from build123d import *

# Parameters (mm, degrees)
F0_W        = 80
F0_H        = 80
F0_R        = 2.5
F0_R_2      = 12
F1_DEPTH    = 2
F2_T1_DEPTH = 90
F2_T3_DEPTH = 90


# Not quite as in the source:
# - a fillet or chamfer that OpenCascade refuses, or shapes differently, is made with other operations: its cross-section is extruded or revolved along the edge and cut away or added


with BuildPart() as f1:
    # F0 (on Front) → F1 (new body)
    with BuildSketch(Plane.XZ):
        with Locations((-0.0017476827, 0.1713572443)):
            Rectangle(F0_W, F0_H)
        with Locations((-36.4662137768, -36.2931088498)):
            Circle(F0_R, mode=Mode.SUBTRACT)
        with Locations((36.4627184114, -36.2931088498)):
            Circle(F0_R, mode=Mode.SUBTRACT)
        with Locations((-36.4662137768, 36.6358233383)):
            Circle(F0_R, mode=Mode.SUBTRACT)
        with BuildLine():
            ThreePointArc((38.4690204407, 1.6713572443), (38.4909436544, 0.9214996478), (38.4982523173, 0.1713572443))
            ThreePointArc((38.4982523173, 0.1713572443), (38.4909464293, -0.5786427557), (38.4690315381, -1.3283581108))
            ThreePointArc((38.4690315381, -1.3283581108), (35.4737380316, -14.7865808935), (27.9287857338, -26.3264785744))
            ThreePointArc((27.9287857338, -26.3264785744), (26.8753996766, -27.3943633128), (25.7812151161, -28.4204043195))
            ThreePointArc((25.7812151161, -28.4204043195), (14.5064210867, -35.4904295724), (1.498122464, -38.2994159419))
            ThreePointArc((1.498122464, -38.2994159419), (0.7484071972, -38.3213338497), (-0.0015927734, -38.3286427554))
            ThreePointArc((-0.0015927734, -38.3286427554), (-0.7517476827, -38.3213368677), (-1.5016178294, -38.2994159419))
            ThreePointArc((-1.5016178294, -38.2994159419), (-14.5093699729, -35.4906518899), (-25.7838341949, -28.421194497))
            ThreePointArc((-25.7838341949, -28.421194497), (-26.8780502008, -27.3951870251), (-27.9314689858, -26.3273345712))
            ThreePointArc((-27.9314689858, -26.3273345712), (-35.4773135858, -14.7863907098), (-38.4725889134, -1.3267665824))
            ThreePointArc((-38.4725889134, -1.3267665824), (-38.4944573001, -0.5778465387), (-38.5017476827, 0.1713572443))
            ThreePointArc((-38.5017476827, 0.1713572443), (-38.4944390198, 0.9214996478), (-38.472515806, 1.6713572443))
            ThreePointArc((-38.472515806, 1.6713572443), (-35.4771780599, 15.1294266234), (-27.9322810992, 26.6691930629))
            ThreePointArc((-27.9322810992, 26.6691930629), (-26.878895042, 27.7370778013), (-25.7847104814, 28.763118808))
            ThreePointArc((-25.7847104814, 28.763118808), (-14.5098447074, 35.8331732485), (-1.5014630377, 38.642136465))
            ThreePointArc((-1.5014630377, 38.642136465), (-0.7517476827, 38.6640513563), (-0.0017476827, 38.6713572443))
            ThreePointArc((-0.0017476827, 38.6713572443), (0.7482523173, 38.6640513563), (1.4979676723, 38.642136465))
            ThreePointArc((1.4979676723, 38.642136465), (14.9561904551, 35.6468429586), (26.4960881359, 28.1018906607))
            ThreePointArc((26.4960881359, 28.1018906607), (27.5639728743, 27.0485046035), (28.5900138811, 25.954320043))
            ThreePointArc((28.5900138811, 25.954320043), (35.6600146487, 14.6795861996), (38.4690204407, 1.6713572443))
        make_face(mode=Mode.SUBTRACT)
        with Locations((36.4627184114, 36.6358233383)):
            Circle(F0_R, mode=Mode.SUBTRACT)
        with BuildLine():
            Line((-9.495982875, 11.7842594703), (-25.7847104814, 28.763118808))
            ThreePointArc((-25.7847104814, 28.763118808), (-26.878895042, 27.7370778013), (-27.9322810992, 26.6691930629))
            Line((-27.9322810992, 26.6691930629), (-11.6157607218, 9.6642335801))
            ThreePointArc((-11.6157607218, 9.6642335801), (-10.608969906, 10.7773384203), (-9.495982875, 11.7842594703))
        make_face()
        with BuildLine():
            ThreePointArc((14.9230924791, -1.3283581108), (14.9794505742, -0.5794415216), (14.9982523173, 0.1713572443))
            ThreePointArc((14.9982523173, 0.1713572443), (14.979443414, 0.9222988702), (14.9230638739, 1.6713572443))
            ThreePointArc((14.9230638739, 1.6713572443), (13.8560844811, 5.9124797581), (11.6111545434, 9.6655924366))
            ThreePointArc((11.6111545434, 9.6655924366), (10.6042334933, 10.7785794675), (9.4911286531, 11.7853702834))
            ThreePointArc((9.4911286531, 11.7853702834), (5.7376930398, 14.0298860332), (1.496376144, 15.0963572443))
            ThreePointArc((1.496376144, 15.0963572443), (0.7482523173, 15.1525955108), (-0.0017476827, 15.1713572443))
            ThreePointArc((-0.0017476827, 15.1713572443), (-0.7517476827, 15.1525955108), (-1.4998715093, 15.0963572443))
            ThreePointArc((-1.4998715093, 15.0963572443), (-5.7419991682, 14.0295502319), (-9.495982875, 11.7842594703))
            ThreePointArc((-9.495982875, 11.7842594703), (-10.608969906, 10.7773384203), (-11.6157607218, 9.6642335801))
            ThreePointArc((-11.6157607218, 9.6642335801), (-13.8599156987, 5.9116690162), (-14.9265592393, 1.6713572443))
            ThreePointArc((-14.9265592393, 1.6713572443), (-14.9829387793, 0.9222988702), (-15.0017476827, 0.1713572443))
            ThreePointArc((-15.0017476827, 0.1713572443), (-14.9829859493, -0.5786427557), (-14.9267476827, -1.3267665824))
            ThreePointArc((-14.9267476827, -1.3267665824), (-13.8599406704, -5.5688942412), (-11.6146499088, -9.3228779481))
            ThreePointArc((-11.6146499088, -9.3228779481), (-10.6083494005, -10.4352444735), (-9.495982875, -11.4415449818))
            ThreePointArc((-9.495982875, -11.4415449818), (-5.7428099115, -13.6864998947), (-1.5016178294, -14.7534673625))
            ThreePointArc((-1.5016178294, -14.7534673625), (-0.7525467792, -14.8098409961), (-0.0015927734, -14.8286427549))
            ThreePointArc((-0.0015927734, -14.8286427549), (0.7492061289, -14.8098332416), (1.498122464, -14.7534673625))
            ThreePointArc((1.498122464, -14.7534673625), (5.7393145462, -13.6864998947), (9.4924875096, -11.4415449818))
            ThreePointArc((9.4924875096, -11.4415449818), (10.6054745406, -10.4346239318), (11.6122653564, -9.3215190916))
            ThreePointArc((11.6122653564, -9.3215190916), (13.8564750721, -5.5688223766), (14.9230924791, -1.3283581108))
        make_face()
        with Locations((-0.0017476827, 0.1713572443)):
            Circle(F0_R_2, mode=Mode.SUBTRACT)
        with BuildLine():
            Line((-0.0017476827, 15.1713572443), (-0.0017476827, 38.6713572443))
            ThreePointArc((-0.0017476827, 38.6713572443), (-0.7517476827, 38.6640513563), (-1.5014630377, 38.642136465))
            Line((-1.5014630377, 38.642136465), (-1.4998715093, 15.0963572443))
            ThreePointArc((-1.4998715093, 15.0963572443), (-0.7517476827, 15.1525955108), (-0.0017476827, 15.1713572443))
        make_face()
        with BuildLine():
            Line((1.496376144, 15.0963572443), (1.4979676723, 38.642136465))
            ThreePointArc((1.4979676723, 38.642136465), (0.7482523173, 38.6640513563), (-0.0017476827, 38.6713572443))
            Line((-0.0017476827, 38.6713572443), (-0.0017476827, 15.1713572443))
            ThreePointArc((-0.0017476827, 15.1713572443), (0.7482523173, 15.1525955108), (1.496376144, 15.0963572443))
        make_face()
        with BuildLine():
            Line((11.6111545434, 9.6655924366), (28.5900138811, 25.954320043))
            ThreePointArc((28.5900138811, 25.954320043), (27.5639728743, 27.0485046035), (26.4960881359, 28.1018906607))
            Line((26.4960881359, 28.1018906607), (9.4911286531, 11.7853702834))
            ThreePointArc((9.4911286531, 11.7853702834), (10.6042334933, 10.7785794675), (11.6111545434, 9.6655924366))
        make_face()
        with BuildLine():
            Line((14.9982523173, 0.1713572443), (38.4982523173, 0.1713572443))
            ThreePointArc((38.4982523173, 0.1713572443), (38.4909436544, 0.9214996478), (38.4690204407, 1.6713572443))
            Line((38.4690204407, 1.6713572443), (14.9230638739, 1.6713572443))
            ThreePointArc((14.9230638739, 1.6713572443), (14.979443414, 0.9222988702), (14.9982523173, 0.1713572443))
        make_face()
        with BuildLine():
            ThreePointArc((38.4690315381, -1.3283581108), (38.4909464293, -0.5786427557), (38.4982523173, 0.1713572443))
            Line((38.4982523173, 0.1713572443), (14.9982523173, 0.1713572443))
            ThreePointArc((14.9982523173, 0.1713572443), (14.9794505742, -0.5794415216), (14.9230924791, -1.3283581108))
            Line((14.9230924791, -1.3283581108), (38.4690315381, -1.3283581108))
        make_face()
        with BuildLine():
            ThreePointArc((25.7812151161, -28.4204043195), (26.8753996766, -27.3943633128), (27.9287857338, -26.3264785744))
            Line((27.9287857338, -26.3264785744), (11.6122653564, -9.3215190916))
            ThreePointArc((11.6122653564, -9.3215190916), (10.6054745406, -10.4346239318), (9.4924875096, -11.4415449818))
            Line((9.4924875096, -11.4415449818), (25.7812151161, -28.4204043195))
        make_face()
        with BuildLine():
            ThreePointArc((-0.0015927734, -38.3286427554), (0.7484071972, -38.3213338497), (1.498122464, -38.2994159419))
            Line((1.498122464, -38.2994159419), (1.498122464, -14.7534673625))
            ThreePointArc((1.498122464, -14.7534673625), (0.7492061289, -14.8098332416), (-0.0015927734, -14.8286427549))
            Line((-0.0015927734, -14.8286427549), (-0.0015927734, -38.3286427554))
        make_face()
        with BuildLine():
            ThreePointArc((-1.5016178294, -38.2994159419), (-0.7517476827, -38.3213368677), (-0.0015927734, -38.3286427554))
            Line((-0.0015927734, -38.3286427554), (-0.0015927734, -14.8286427549))
            ThreePointArc((-0.0015927734, -14.8286427549), (-0.7525467792, -14.8098409961), (-1.5016178294, -14.7534673625))
            Line((-1.5016178294, -14.7534673625), (-1.5016178294, -38.2994159419))
        make_face()
        with BuildLine():
            ThreePointArc((-27.9314689858, -26.3273345712), (-26.8780502008, -27.3951870251), (-25.7838341949, -28.421194497))
            Line((-25.7838341949, -28.421194497), (-9.495982875, -11.4415449818))
            ThreePointArc((-9.495982875, -11.4415449818), (-10.6083494005, -10.4352444735), (-11.6146499088, -9.3228779481))
            Line((-11.6146499088, -9.3228779481), (-27.9314689858, -26.3273345712))
        make_face()
        with BuildLine():
            ThreePointArc((-38.5017476827, 0.1713572443), (-38.4944573001, -0.5778465387), (-38.4725889134, -1.3267665824))
            Line((-38.4725889134, -1.3267665824), (-14.9267476827, -1.3267665824))
            ThreePointArc((-14.9267476827, -1.3267665824), (-14.9829859493, -0.5786427557), (-15.0017476827, 0.1713572443))
            Line((-15.0017476827, 0.1713572443), (-38.5017476827, 0.1713572443))
        make_face()
        with BuildLine():
            Line((-14.9265592393, 1.6713572443), (-38.472515806, 1.6713572443))
            ThreePointArc((-38.472515806, 1.6713572443), (-38.4944390198, 0.9214996478), (-38.5017476827, 0.1713572443))
            Line((-38.5017476827, 0.1713572443), (-15.0017476827, 0.1713572443))
            ThreePointArc((-15.0017476827, 0.1713572443), (-14.9829387793, 0.9222988702), (-14.9265592393, 1.6713572443))
        make_face()
    extrude(amount=F1_DEPTH)

    # F2: fillet of radius 2 on 5 edges, made by hand

    # F2_s2 → F2_t1 (cut)
    with BuildSketch(Plane.YZ.offset(-45.0017476827)):
        with BuildLine():
            ThreePointArc((0, 40.1713572443), (-1.4142135624, 39.5855708066), (-2, 38.1713572443))
            Line((-2, 38.1713572443), (-2, 40.1713572443))
            Line((-2, 40.1713572443), (0, 40.1713572443))
        make_face()
        with BuildLine():
            ThreePointArc((0, -39.8286427557), (-1.4142135624, -39.2428563181), (-2, -37.8286427557))
            Line((-2, -37.8286427557), (-2, -39.8286427557))
            Line((-2, -39.8286427557), (0, -39.8286427557))
        make_face()
    extrude(amount=F2_T1_DEPTH, mode=Mode.SUBTRACT)

    # F2_s4 → F2_t3 (cut)
    with BuildSketch(Plane.XY.offset(-44.8286427557)):
        with BuildLine():
            ThreePointArc((39.9982523173, 0), (39.4124658797, -1.4142135624), (37.9982523173, -2))
            Line((37.9982523173, -2), (39.9982523173, -2))
            Line((39.9982523173, -2), (39.9982523173, 0))
        make_face()
        with BuildLine():
            ThreePointArc((-40.0017476827, 0), (-39.4159612451, -1.4142135624), (-38.0017476827, -2))
            Line((-38.0017476827, -2), (-40.0017476827, -2))
            Line((-40.0017476827, -2), (-40.0017476827, 0))
        make_face()
    extrude(amount=F2_T3_DEPTH, mode=Mode.SUBTRACT)

    # F2_s5 → F2_t6 (revolve, cut)
    with BuildSketch(Plane.XY.offset(0.1713572443)):
        with BuildLine():
            ThreePointArc((11.9982523173, 0), (12.5840387549, -1.4142135624), (13.9982523173, -2))
            Line((13.9982523173, -2), (11.9982523173, -2))
            Line((11.9982523173, -2), (11.9982523173, 0))
        make_face()
    revolve(axis=Axis((-0.0017476827, -2, 0.1713572443), (0, -1, 0)), mode=Mode.SUBTRACT)


solid = f1.part
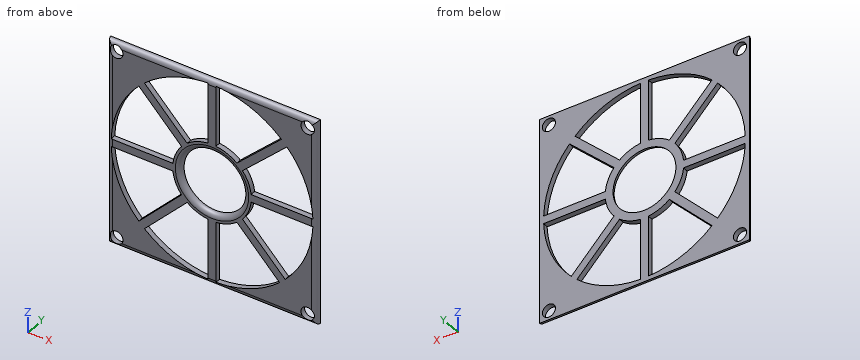
Check sheet for the modelled part. Datum: model origin and axes. Units: mm. Round coordinates to 2 decimals unless told otherwise and drop trailing zeros. Loops run counter-clockwise (first coordinate to the right, second up) from the corner with the lowest first, then second, coordinate; pieces in that order, holes last. Notation, with made-up numbers: M 59.5,71 L 92.5,71 A21 cw 92.5,105 Z; hole C -36,-29.75 d4. An arc over 180 degrees is marked long. One line per item, written item: value.
(1) Thickness scan on line 1 (X direction, y = -1.2, z = -22); line 2 (X direction, y = -0.85, z = -31); line 3 (X direction, y = -1.6, z = 27). Record the ranges inside material, lowest first.
Computed values:
line 1: x = -39.6 to -31.48, -23.78 to -19.62, -1.5 to 1.5, 19.62 to 23.78, 31.47 to 39.6
line 2: x = -39.81 to -22.6, -1.5 to 1.5, 22.59 to 39.81
line 3: x = -39.2 to -24.09, -1.5 to 1.5, 25.35 to 39.2
(2) Sectioned sample at A-A, the plane x = 23.5. Record the cut outline in (y, z).
Computed values:
outline: M -2,-37.83 A2 ccw 0,-39.83 L 0,-30.32 L -2,-30.32 Z; M -2,-26.04 L 0,-26.04 L 0,-21.71 L -2,-21.71 Z; M -2,-1.33 L 0,-1.33 L 0,1.67 L -2,1.67 Z; M -2,21.07 L 0,21.07 L 0,25.23 L -2,25.23 Z; M -2,30.67 L 0,30.67 L 0,40.17 A2 ccw -2,38.17 Z
(3) Sectioned sample at D-D, the plane y = -0.65. Count the separate pieces of the cut face and the enclosed holes in it, then the cut area to 3 significant figures.
Computed values:
separate pieces: 1
enclosed holes: 13
area: 2,440 mm^2
(4) Sectioned sample at B-B, the plane z = -22. Record the cut outline in (x, y).
Computed values:
outline: M -40,0 A2 ccw -38,-2 L -31.48,-2 L -31.48,0 Z; M -23.78,-2 L -19.62,-2 L -19.62,0 L -23.78,0 Z; M -1.5,-2 L 1.5,-2 L 1.5,0 L -1.5,0 Z; M 19.62,-2 L 23.78,-2 L 23.78,0 L 19.62,0 Z; M 31.47,-2 L 38,-2 A2 ccw 40,0 L 31.47,0 Z
(5) Depth check by flat-ended pin: pin 1 Ø0.6 at (y, z) = (-1.5, -30.5) entering from +X; pin 2 Ø4.5 at (x, z) = (-36.47, 36.64) entering from -Y; pin 3 Ø0.6 at (y, z) = (-1, -22) entering from -X; pin 4 Ø0.6 at (x, y) = (21.5, -0.5) entering from -Z. Enter the tip coordinate at first touch or a pass-through.
Computed values:
pin 1: stops at x = 39.6
pin 2: passes through
pin 3: stops at x = -39.88
pin 4: stops at z = -39.82
(6) Sectioned sample at C-C, the plane x = -32. Record the cut outline in (y, z), then the cut area to 3 significant figures.
Computed values:
outline: M -2,-37.83 A2 ccw 0,-39.83 L 0,-21.24 L -2,-21.24 Z; M -2,-1.33 L 0,-1.33 L 0,1.67 L -2,1.67 Z; M -2,21.58 L 0,21.58 L 0,40.17 A2 ccw -2,38.17 Z
area: 78.6 mm^2
